Part model, mm, in its own coordinate system. A direction names the side the tool comes from. Give positions to 0.01 mm unless a question says otherwise; leave off trailing zeros. Loops run counter-clockwise (first coordinate to the right, second up) from the corner with the lowest first, then second, coordinate; pieces in that order, holes last. Notation, with made-up numbers: M 69.25,-37 L 113.25,-37 A12 ccw 113.25,-21 Z; hole C 40,82.5 d1. An arc over 180 degrees is marked long. Answer in a Markdown table with one row per item.
from build123d import *

# Parameters (mm, degrees)
EXTRUDE_1_DEPTH     = 5.5
SKETCH_2_R          = 2
CUT_EXTRUDE_1_DEPTH = 10.014432872
FILLET_1_R          = 0.4


with BuildPart() as part:
    # 草图1 → 凸台-拉伸1 (new, symmetric)
    with BuildSketch(Plane.XY):
        Polygon((-5.1, 0), (-3, 0), (-3, 1), (3, 1), (3, 0), (5.1, 0), (5.1, -1.9), (3, -4), (-3, -4), (-5.1, -1.9), align=None)
    extrude(amount=EXTRUDE_1_DEPTH, both=True)

    # 草图2 → 切除-拉伸1 (cut, through all)
    with BuildSketch(Plane(origin=(0, 1, 0), x_dir=(1, 0, 0), z_dir=(0, 1, 0))):
        with Locations(Location((0, 0, 0), (0, 0, 270))):
            Circle(SKETCH_2_R)
    extrude(amount=-CUT_EXTRUDE_1_DEPTH, mode=Mode.SUBTRACT)

    # 圆角1
    fillet_1_edges = [part.edges().sort_by_distance(p)[0] for p in [
        (-5.1, 0, 0),
        (-3, 1, 0),
        (3, 1, 0),
        (5.1, 0, 0),
        (5.1, -1.9, 0),
        (3, -4, 0),
        (-3, -4, 0),
        (-5.1, -1.9, 0),
    ]]
    fillet(fillet_1_edges, radius=FILLET_1_R)


solid = part.part
(1) Pin check, flat tips, straight feed: pin 1 Ø0.8 at (x, z) = (4, 0) entering from +Y; pin 2 Ø0.7 at (y, z) = (0, -2) entering from -X. Stop position of each tip, or through.
Recorded:
| item | result |
|---|---|
| pin 1 | stops at y = 0 |
| pin 2 | stops at x = -5.1 |
(2) Which spindle directions (+Z, -Z, +X, -X, +Y, -Y) get a long thin tool onto all of the face, cutting with end or side? Do faces 5 (the face through (-2, 1, -1)), 6 (the face through (4, 0, 0)). Say none if no direction does.
Recorded:
| item | result |
|---|---|
| face 5 | +Z, -Z, +X, -X, +Y |
| face 6 | +Z, -Z, +X, +Y |
(3) Saw through at A-A (z = 0). Write the cut outline in (x, y), plus the area to 3 significant figures.
Recorded:
| item | result |
|---|---|
| outline | M -5.1,-1.73 A0.4 ccw -4.98,-2.02 L -3.12,-3.88 A0.4 ccw -2.83,-4 L -2,-4 L -2,1 L -2.6,1 A0.4 ccw -3,0.6 L -3,0 L -4.7,0 A0.4 ccw -5.1,-0.4 Z; M 2,-4 L 2.83,-4 A0.4 ccw 3.12,-3.88 L 4.98,-2.02 A0.4 ccw 5.1,-1.73 L 5.1,-0.4 A0.4 ccw 4.7,0 L 3,0 L 3,0.6 A0.4 ccw 2.6,1 L 2,1 Z |
| area | 22.2 mm^2 |
(4) Pull direction Z, two halves, no side cores. Call faces 1 (the face through (0, -1, -5.5)), 2 (the face through (-4, 0, 0)), 3 (the face through (0, -1, 5.5)), 4 (the face through (-2, -1, 0)): +Z half, -Z half, draft (parallel to the pull), parting line (faces both ways), or undercut.
Recorded:
| item | result |
|---|---|
| face 1 | -Z half |
| face 2 | draft |
| face 3 | +Z half |
| face 4 | undercut |
(5) Saw through at B-B (x = 0). Write the cut outline in (y, z).
Recorded:
| item | result |
|---|---|
| outline | M -4,-5.5 L 1,-5.5 L 1,-2 L -4,-2 Z; M -4,2 L 1,2 L 1,5.5 L -4,5.5 Z |
(6) Saw through at C-C (y = 0.2). Write the cut outline in (x, z), plus the area to 3 significant figures.
Recorded:
| item | result |
|---|---|
| outline | M -3,-5.5 L 3,-5.5 L 3,5.5 L -3,5.5 Z; hole C 0,0 d4 |
| area | 53.4 mm^2 |
(7) Saw through at D-D (z = 3.75). Write the cut outline in (x, y).
Recorded:
| item | result |
|---|---|
| outline | M -5.1,-1.73 A0.4 ccw -4.98,-2.02 L -3.12,-3.88 A0.4 ccw -2.83,-4 L 2.83,-4 A0.4 ccw 3.12,-3.88 L 4.98,-2.02 A0.4 ccw 5.1,-1.73 L 5.1,-0.4 A0.4 ccw 4.7,0 L 3,0 L 3,0.6 A0.4 ccw 2.6,1 L -2.6,1 A0.4 ccw -3,0.6 L -3,0 L -4.7,0 A0.4 ccw -5.1,-0.4 Z |
(8) Drill centre lines: line 1 along X through (y, z) = (-1.15, 0); line 2 along X through (y, z) = (-2.3, 0); line 3 along Z through (x, y) = (1.75, -2.8). Where is each one in solid material? Low to high.
Recorded:
| item | result |
|---|---|
| line 1 | x = -5.1 to -2, 2 to 5.1 |
| line 2 | x = -4.7 to -2, 2 to 4.7 |
| line 3 | z = -5.5 to -0.97, 0.97 to 5.5 |
